Verification items for this drawing (mm, ordinates from the low corner). A direction names the side the tool comes from. Coordinates: 2 decimals unless noted, no trailing zeros. Order: outer loops, then holes, each group sorted by start corner. A loop starts at its lowest first (then second) coordinate and runs counter-clockwise, first axis right, second up. Notation, with made-up numbers: (41, 62) -> (77, 62) arc R16 ccw to (77, 93) -> close; hole circle Ø9 at (52, 76.25). An arc over 180 degrees is marked (long way). Answer in a Markdown table with one row per item. Add a question column.
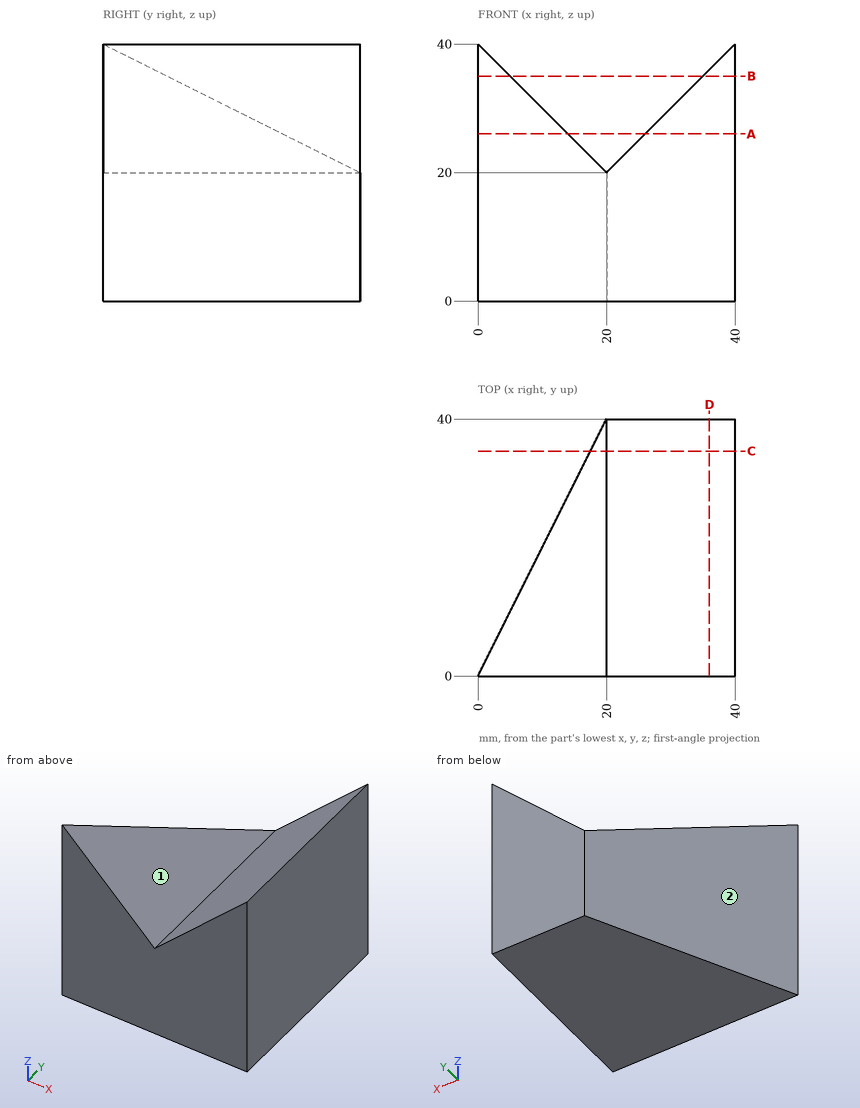
(1) Scan lines: line 1 along Y through (x, z) = (10, 6); line 2 along X through (y, z) = (2, 21); line 3 along X through (y, z) = (34.5, 27.5). Record each from-to range of solid material in increasing order.
(2) Go/stop test with flat-tipped pins: P1, Ø12, axis at x = 5.5, z = 4.5, coming from the +Y side; P2, Ø2, axis at x = 22.5, y = 33, coming from the +Z side; P3, Ø1, axis at x = 9.5, z = 24.5, coming from the +Y side; P4, Ø3, axis at x = 20.5, y = 20.5, coming from the -Z side. Record where each tip stops, or that it passes through.
(3) Cross-section at B-B (z = 35). Enter the section's corners in (x, y), plus the area to 3 significant figures.
(4) Cross-section at D-D (x = 36). Enter the section's corners in (y, z), plus the area to 3 significant figures.
(5) Access from +Z, -Z, +X, -X, +Y, -Y to the whole of each face (thin tool, end or side, straight path). Record for the marked faces 1 and 2.
(6) Cross-section at A-A (z = 26). Enter the section's corners in (x, y), plus the area to 3 significant figures.
(7) Cross-section at C-C (y = 35). Enter the section's corners in (x, z).
Checks:
| question | item | result |
|---|---|---|
| 1 | line 1 | 0 to 20 |
| 1 | line 2 | 1 to 19, 21 to 40 |
| 1 | line 3 | 27.5 to 40 |
| 2 | P1 | y = 23 |
| 2 | P2 | z = 23.5 |
| 2 | P3 | y = 20 |
| 2 | P4 | z = 0 |
| 3 | outline | (0, 0) -> (5, 0) -> (5, 10) -> close; (35, 0) -> (40, 0) -> (40, 40) -> (35, 40) -> close |
| 3 | area | 225 mm² |
| 4 | outline | (0, 0) -> (40, 0) -> (40, 36) -> (0, 36) -> close |
| 4 | area | 1,440 mm² |
| 5 | face 1 | +Z, +Y, -Y |
| 5 | face 2 | +Z, -Z, -X, +Y |
| 6 | outline | (0, 0) -> (14, 0) -> (14, 28) -> close; (26, 0) -> (40, 0) -> (40, 40) -> (26, 40) -> close |
| 6 | area | 756 mm² |
| 7 | outline | (17.5, 0) -> (40, 0) -> (40, 40) -> (20, 20) -> (17.5, 22.5) -> close |
